For this review, take the finished solid that the model builds, in its own axes (mm). Face numbers are marked on the shaded views. A direction names the side the tool comes from. Round coordinates to 2 decimals unless told otherwise and drop trailing zeros. Write each loop counter-clockwise with the first axis right and the second up, starting at its lowest first coordinate (ties: lowest second). Pieces come first, ordered by that corner, then holes. Notation, with made-up numbers: (-21, -16.75) -> (-6, -16.75) arc R29 ccw to (-6, 4.25) -> close; hole circle Ø5 at (41, -27.5). An arc over 180 degrees is marked (long way). Answer in a Markdown table with one row per item.
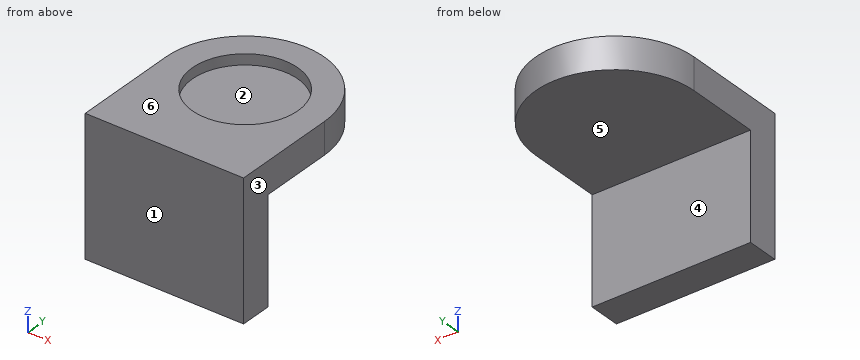
from build123d import *

# Parameters (mm, degrees)
SKETCH6_R           = 5
BOSS_EXTRUDE5_DEPTH = 3
SKETCH7_R           = 5
BOSS_EXTRUDE6_DEPTH = 2
SKETCH8_W           = 15
SKETCH8_H           = 3
BOSS_EXTRUDE7_DEPTH = 10


with BuildPart() as part:
    # Sketch6 → Boss-Extrude5 (new body)
    with BuildSketch(Plane.XY):
        with BuildLine():
            Line((-7.5, 0), (-7.5, -10))
            Line((-7.5, -10), (7.5, -10))
            Line((7.5, -10), (7.5, 0))
            ThreePointArc((7.5, 0), (0, 7.5), (-7.5, 0))
        make_face()
        Circle(SKETCH6_R, mode=Mode.SUBTRACT)
    extrude(amount=BOSS_EXTRUDE5_DEPTH)

    # Sketch7 → Boss-Extrude6 (add)
    with BuildSketch(Plane(origin=(0, 0, 0), x_dir=(-1, 0, 0), z_dir=(0, 0, -1))):
        Circle(SKETCH7_R)
    extrude(amount=-BOSS_EXTRUDE6_DEPTH)

    # Sketch8 → Boss-Extrude7 (add)
    with BuildSketch(Plane(origin=(0, 0, 0), x_dir=(-1, 0, 0), z_dir=(0, 0, -1))):
        with Locations((0, -8.5)):
            Rectangle(SKETCH8_W, SKETCH8_H)
    extrude(amount=BOSS_EXTRUDE7_DEPTH)


solid = part.part
1) For the marked faces 5 and 6, list the 3-axis set-ups (+Z, -Z, +X, -X, +Y, -Y) from which the entire face can be reached by the end or side of a thin tool; tool diameter is ignored.
Solved:
| item | result |
|---|---|
| face 5 | -Z, +X, -X, +Y |
| face 6 | +Z, +X, -X, +Y, -Y |
2) Consider section C-C on z = 0.25. State the section outline as (x, y) points.
Solved:
| item | result |
|---|---|
| outline | (-7.5, -10) -> (7.5, -10) -> (7.5, 0) arc R7.5 ccw to (-7.5, 0) -> close |
3) Clearance check with flat-ended pins moving along their axes: pin 1 Ø2 at (y, z) = (-4, -2.5) entering from +X; pin 2 Ø1.5 at (x, z) = (-0.5, -1) entering from +Y; pin 3 Ø7 at (x, y) = (1.5, -0.5) entering from -Z. State where each tip first meets the part, or that it passes through.
Solved:
| item | result |
|---|---|
| pin 1 | through |
| pin 2 | y = -7 |
| pin 3 | z = 0 |
4) Mouldability with a two-part tool opening along Y and no side actions: class the marked faces 1, 2, 3 and 4 as pulls with the +Y half, pulls with the -Y half, needs draft (parallel to the pull), parting line crosses it, or undercut.
Solved:
| item | result |
|---|---|
| face 1 | pulls with the -Y half |
| face 2 | undercut |
| face 3 | needs draft |
| face 4 | pulls with the +Y half |
5) Consider section A-A on x = 6. State the section outline as (y, z) points.
Solved:
| item | result |
|---|---|
| outline | (-10, -10) -> (-7, -10) -> (-7, 0) -> (4.5, 0) -> (4.5, 3) -> (-10, 3) -> close |
6) Consider section B-B on y = 1.25. State the section outline as (x, z) points.
Solved:
| item | result |
|---|---|
| outline | (-7.4, 0) -> (7.4, 0) -> (7.4, 3) -> (4.84, 3) -> (4.84, 2) -> (-4.84, 2) -> (-4.84, 3) -> (-7.4, 3) -> close |
7) Consider section D-D on x = 0.75. State the section outline as (y, z) points, then the cut area to 3 significant figures.
Solved:
| item | result |
|---|---|
| outline | (-10, -10) -> (-7, -10) -> (-7, 0) -> (7.46, 0) -> (7.46, 3) -> (4.94, 3) -> (4.94, 2) -> (-4.94, 2) -> (-4.94, 3) -> (-10, 3) -> close |
| area | 72.5 mm² |
8) For line 1 (Y direction, x = 0, z = 2.8); line 2 (Z direction, x = 4.25, y = 0.25); line 3 (Z direction, x = 6, y = 2.25), list the stretches that pass through material, from the lowest coordinate up. Write a range as [from, to].
Solved:
| item | result |
|---|---|
| line 1 | [-10, -5], [5, 7.5] |
| line 2 | [0, 2] |
| line 3 | [0, 3] |
